from build123d import *

# Parameters (mm, degrees)
SKETCH1_W           = 69.85
SKETCH1_H           = 95.25
BOSS_EXTRUDE1_DEPTH = 28.575
FILLET1_R           = 12.7
SKETCH2_OUTSIDE_W   = 96.154
SKETCH2_OUTSIDE_H   = 121.554
SKETCH2_OUTSIDE_R   = 5.715
CUT_EXTRUDE1_DEPTH  = 4.064


with BuildPart() as part:
    # Sketch1 → Boss-Extrude1 (new body)
    with BuildSketch(Plane.XY):
        with Locations((34.925, 47.625)):
            Rectangle(SKETCH1_W, SKETCH1_H)
    extrude(amount=BOSS_EXTRUDE1_DEPTH)

    # Fillet1
    fillet1_edges = [part.edges().sort_by_distance(p)[0] for p in [
        (0, 95.25, 14.2875),
        (69.85, 95.25, 14.2875),
        (69.85, 0, 14.2875),
        (0, 0, 14.2875),
    ]]
    fillet(fillet1_edges, radius=FILLET1_R)

    # Sketch2 outside → Cut-Extrude1 (cut)
    # profile 1 of 3: a face of its own
    with BuildSketch(Plane.XY.offset(28.575)):
        with Locations((34.925, 47.625)):
            Rectangle(SKETCH2_OUTSIDE_W, SKETCH2_OUTSIDE_H)
        with Locations((60.96, 8.89)):
            Circle(SKETCH2_OUTSIDE_R, mode=Mode.SUBTRACT)
        with Locations((8.89, 8.89)):
            Circle(SKETCH2_OUTSIDE_R, mode=Mode.SUBTRACT)
        with Locations((8.89, 86.36)):
            Circle(SKETCH2_OUTSIDE_R, mode=Mode.SUBTRACT)
        with Locations((60.96, 86.36)):
            Circle(SKETCH2_OUTSIDE_R, mode=Mode.SUBTRACT)
        with BuildLine():
            Line((37.7825, 6.35), (32.0675, 6.35))
            ThreePointArc((32.0675, 6.35), (26.9875, 11.43), (32.0675, 16.51))
            Line((32.0675, 16.51), (37.7825, 16.51))
            ThreePointArc((37.7825, 16.51), (42.8625, 11.43), (37.7825, 6.35))
        make_face(mode=Mode.SUBTRACT)
        with BuildLine():
            Line((37.7825, 78.74), (32.0675, 78.74))
            ThreePointArc((32.0675, 78.74), (26.9875, 83.82), (32.0675, 88.9))
            Line((32.0675, 88.9), (37.7825, 88.9))
            ThreePointArc((37.7825, 88.9), (42.8625, 83.82), (37.7825, 78.74))
        make_face(mode=Mode.SUBTRACT)
    # profile 2 of 3: a face of its own
    with BuildSketch(Plane.XY.offset(28.575)):
        with BuildLine():
            Line((32.0675, 14.77282006), (34.301719909, 14.77282006))
            ThreePointArc((34.301719909, 14.77282006), (42.6085, 11.43), (34.301719909, 8.08717994))
            Line((34.301719909, 8.08717994), (32.0675, 8.08717994))
            ThreePointArc((32.0675, 8.08717994), (28.72467994, 11.43), (32.0675, 14.77282006))
        make_face()
    # profile 3 of 3: a face of its own
    with BuildSketch(Plane.XY.offset(28.575)):
        with BuildLine():
            Line((32.0675, 80.47717994), (34.301719909, 80.47717994))
            ThreePointArc((34.301719909, 80.47717994), (42.6085, 83.82), (34.301719909, 87.16282006))
            Line((34.301719909, 87.16282006), (32.0675, 87.16282006))
            ThreePointArc((32.0675, 87.16282006), (28.72467994, 83.82), (32.0675, 80.47717994))
        make_face()
    extrude(amount=-CUT_EXTRUDE1_DEPTH, mode=Mode.SUBTRACT)


solid = part.part
Here's how the part is built. I have some questions about the finished solid (model axes, mm). A direction names the side the tool comes from. Round coordinates to 2 decimals unless told otherwise and drop trailing zeros. Order: outer loops, then holes, each group sorted by start corner. A loop starts at its lowest first (then second) coordinate and runs counter-clockwise, first axis right, second up. Notation, with made-up numbers: M 26,74 L 44,74 A36 cw 44,113 Z; hole C -11,42.5 d5. An arc over 180 degrees is marked long. One line per question, with ' | ' between items.
1) I'm going to push flat-ended pins straight in: pin 1 Ø5 at (x, y) = (16.5, 63) entering from +Z; pin 2 Ø1.8 at (x, z) = (32.5, 26.5) entering from -Y; pin 3 Ø3.5 at (x, z) = (34.5, 27.5) entering from +Y. Where does each tip first touch, or does it pass through?
Checked values:
pin 1: stops at z = 24.51 | pin 2: stops at y = 6.35 | pin 3: stops at y = 88.9
2) Imagine slicing it at D-D, the plane x = 60.96. Write out the boundary of the cut face in (y, z) (3 decimals).
Checked values:
outline: M 0.585,0 L 94.665,0 L 94.665,24.511 L 92.075,24.511 L 92.075,28.575 L 80.645,28.575 L 80.645,24.511 L 14.605,24.511 L 14.605,28.575 L 3.175,28.575 L 3.175,24.511 L 0.585,24.511 Z
3) On a 3-axis mill with a long thin cutter (end or side, diameter ignored), from which of +Z, -Z, +X, -X, +Y, -Y can I reach the whole of each face in a straight line? I mean faces 3 (the flat face through (35, 88.9, 27)), 4 (the flat face through (35, 6.35, 27)), 5 (the flat face through (9, 9, 28.575)), 6 (the flat face through (34, 48, 0)), 7 (the cylindrical face through (26.99, 11.32, 26.57)). Say none if no direction works.
Checked values:
face 3: +Z, +Y | face 4: +Z, -Y | face 5: +Z, +X, -X, +Y, -Y | face 6: -Z, +X, -X, +Y, -Y | face 7: +Z
4) Imagine slicing it at A-A, the plane z = 10.5. Write out the boundary of the cut face in (x, y), plus the area to 3 significant figures.
Checked values:
outline: M 0,12.7 A12.7 ccw 12.7,0 L 57.15,0 A12.7 ccw 69.85,12.7 L 69.85,82.55 A12.7 ccw 57.15,95.25 L 12.7,95.25 A12.7 ccw 0,82.55 Z | area: 6,510 mm²
5) We'd pull the mould along X, two halves only. Please class faces 1 (the flat face through (35, 78.74, 27)), 2 (the flat face through (33, 14.773, 27)): released by +X, released by -X, zero draft, split by the parting line, or undercut.
Checked values:
face 1: zero draft | face 2: undercut
6) Imagine slicing it at B-B, the plane x = 39.5. Write out the boundary of the cut face in (y, z) (3 decimals), plus the area to 3 significant figures.
Checked values:
outline: M 0,0 L 95.25,0 L 95.25,24.511 L 88.601,24.511 L 88.601,28.575 L 88.33,28.575 L 88.33,24.511 L 79.31,24.511 L 79.31,28.575 L 79.039,28.575 L 79.039,24.511 L 16.211,24.511 L 16.211,28.575 L 15.94,28.575 L 15.94,24.511 L 6.92,24.511 L 6.92,28.575 L 6.649,28.575 L 6.649,24.511 L 0,24.511 Z | area: 2,340 mm²
7) I need wall thicknesses on line 1 (X direction, y = 83.82, z = 27.5); line 2 (Y direction, x = 61, z = 25.5); line 3 (Z direction, x = 20, y = 64.5). Which ranges of each line are inside material? Lowest first, please.
Checked values:
line 1: x = 3.77 to 14.01, 26.99 to 28.72, 42.61 to 42.86, 55.84 to 66.08 | line 2: y = 3.18 to 14.6, 80.65 to 92.07 | line 3: z = 0 to 24.51
